Can you work these out from the model? Positions are in its coordinate system, mm. Give positions to 0.01 mm unless a question says otherwise; leave off trailing zeros. Write each loop counter-clockwise with the first axis right and the second up, starting at its lowest first coordinate (ties: lowest second). Pieces come first, ordered by that corner, then holes. Notation, with made-up numbers: (-31.5, 43.5) -> (8.5, 43.5) arc R18 ccw to (8.5, 54.5) -> close; hole circle Ø4 at (15, 35.5). An arc over 180 degrees is marked (long way). One line per item, written item: value.
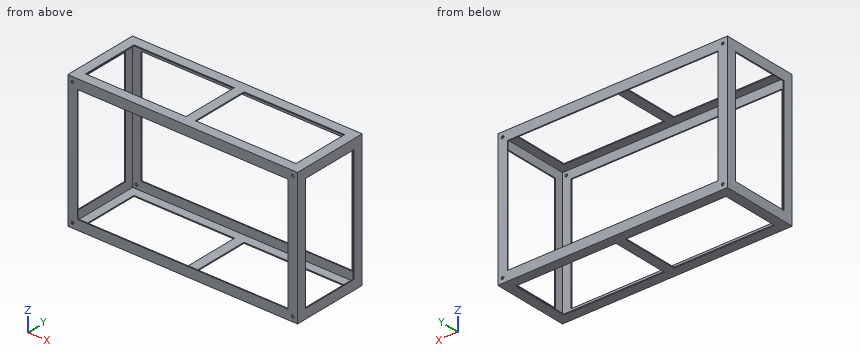
from build123d import *

# Parameters (mm, degrees)
SKETCH8_W           = 50
SKETCH8_H           = 300
BOSS_EXTRUDE2_DEPTH = 5
BOSS_EXTRUDE3_DEPTH = 600
SKETCH11_R          = 7
CUT_EXTRUDE1_DEPTH  = 405


with BuildPart() as part:
    # Sweep1: sweep along a path in Sketch3
    with BuildLine(Plane.XY) as sweep1_path:
        Line((0, 0), (1200, 0))
        Line((1200, 0), (1200, -400))
        Line((1200, -400), (0, -400))
        Line((0, -400), (0, 0))
    # Sketch1 → Sweep1 (sweep)
    with BuildSketch(Plane(origin=(0, 0, 0), x_dir=(0, 0, -1), z_dir=(1, 0, 0))):
        Polygon((0, 0), (0, -50), (5, -50), (5, -5), (50, -5), (50, 0), align=None)
    sweep(path=sweep1_path.line, transition=Transition.RIGHT)

    # Sketch8 → Boss-Extrude2 (add)
    with BuildSketch(Plane.XY):
        with Locations((600, -200)):
            Rectangle(SKETCH8_W, SKETCH8_H)
    extrude(amount=-BOSS_EXTRUDE2_DEPTH)


with BuildPart() as body_2:
    # Mirror8: mirrored copy
    add(part.part.mirror(Plane.XY.offset(-350)))


with BuildPart() as part_1:
    add(part.part)

    add(body_2.part)  # Boss-Extrude3 merges body 2
    # Sketch10 → Boss-Extrude3 (add)
    with BuildSketch(Plane.XY.offset(-650)):
        Polygon((50, 0), (0, 0), (0, -50), (5, -50), (5, -5), (50, -5), align=None)
        Polygon((1195, -50), (1200, -50), (1200, 0), (1150, 0), (1150, -5), (1195, -5), align=None)
        Polygon((1150, -400), (1200, -400), (1200, -350), (1195, -350), (1195, -395), (1150, -395), align=None)
        Polygon((5, -350), (0, -350), (0, -400), (50, -400), (50, -395), (5, -395), align=None)
    extrude(amount=BOSS_EXTRUDE3_DEPTH)

    # Sketch11 → Cut-Extrude1 (cut)
    with BuildSketch(Plane.XZ.offset(400)):
        with Locations(Location((25, -25, 0), (0, 0, 270))):
            Circle(SKETCH11_R)
        with Locations(Location((1175, -25, 0), (0, 0, 270))):
            Circle(SKETCH11_R)
        with Locations(Location((1175, -675, 0), (0, 0, 270))):
            Circle(SKETCH11_R)
        with Locations(Location((25, -675, 0), (0, 0, 270))):
            Circle(SKETCH11_R)
    extrude(amount=-CUT_EXTRUDE1_DEPTH, mode=Mode.SUBTRACT)


solid = part_1.part
1) If we section it at C-C (z = -276): Write out the boundary of the cut face in (x, y).
Answer list:
outline: (0, -400) -> (50, -400) -> (50, -395) -> (5, -395) -> (5, -350) -> (0, -350) -> close; (0, -50) -> (5, -50) -> (5, -5) -> (50, -5) -> (50, 0) -> (0, 0) -> close; (1150, -400) -> (1200, -400) -> (1200, -350) -> (1195, -350) -> (1195, -395) -> (1150, -395) -> close; (1150, -5) -> (1195, -5) -> (1195, -50) -> (1200, -50) -> (1200, 0) -> (1150, 0) -> close
2) I need wall thicknesses on L1, parallel to Z at x = 1175, y = -397; L2, parallel to X at y = -397.2, z = -675; L3, parallel to Z at x = 721, y = -361. Which ranges of each line are inside material? Lowest first, please.
Answer list:
L1: z = -700 to -682, -668 to -32, -18 to 0
L2: x = 0 to 18, 32 to 1168, 1182 to 1200
L3: z = -700 to -695, -5 to 0
3) If we section it at A-A (y = -176): State how many separate pieces and enclosed holes the cut face has, and give its area (3 significant figures).
Answer list:
separate pieces: 6
enclosed holes: 0
area: 2,400 mm^2
4) If we section it at B-B (x = 525.5): Write out the boundary of the cut face in (y, z).
Answer list:
outline: (-400, -700) -> (-350, -700) -> (-350, -695) -> (-395, -695) -> (-395, -650) -> (-400, -650) -> close; (-400, -50) -> (-395, -50) -> (-395, -5) -> (-350, -5) -> (-350, 0) -> (-400, 0) -> close; (-50, -700) -> (0, -700) -> (0, -650) -> (-5, -650) -> (-5, -695) -> (-50, -695) -> close; (-50, -5) -> (-5, -5) -> (-5, -50) -> (0, -50) -> (0, 0) -> (-50, 0) -> close
